Autodesk Inventor part; units mm, degrees
ref_plane "YZ Plane" through (0, 0, 0) normal (1, 0, 0) x (0, 1, 0)
ref_plane "XZ Plane" through (0, 0, 0) normal (0, 1, 0) x (-1, 0, 0)
ref_plane "XY Plane" through (0, 0, 0) normal (0, 0, 1) x (1, 0, 0)
sketch "Esquisse1" plane through (0, 0, 0) normal (0, 1, 0) x (-1, 0, 0)
  circle A0 centre (0, 0) radius 12.5
  dimension "d0" = 25
extrude "Extrusion1" add sketch "Esquisse1" along normal blind 2
sketch "Esquisse2" plane through (0, 2, 0) normal (0, 1, 0) x (1, 0, 0)
  circle A0 centre (0, 0) radius 12.5
  circle A1 centre (0, 0) radius 3.5
  dimension "d3" = 7
extrude "Extrusion2" add sketch "Esquisse2" along normal blind 2 contours A1
sketch "Esquisse3" plane through (0, 4, 0) normal (0, 1, 0) x (1, 0, 0)
  circle A0 centre (0, 0) radius 3.5
  circle A1 centre (0, 0) radius 1.5
  line L0 (-1.118, -1) -> (1.118, -1)
  dimension "d6" = 3
  dimension "d7" = 2.5
extrude "Extrusion3" cut sketch "Esquisse3" against normal through all contours A1 L0 picked at (0.0594, -0.1702)
properties part number "Poulie2"
Geometry check sheet. Reference: the model listing, model coordinates, mm. A direction names the side the tool comes from. Round coordinates to 2 decimals unless told otherwise and drop trailing zeros. Write each loop counter-clockwise with the first axis right and the second up, starting at its lowest first coordinate (ties: lowest second). Pieces come first, ordered by that corner, then holes.
Item 1: Go/stop test with flat-tipped pins: pin 1 Ø0.7 at (x, y) = (0, 3) entering from -Z; pin 2 Ø2 at (x, y) = (3.5, 1.5) entering from -Z; pin 3 Ø1.5 at (y, z) = (2.5, 5.5) entering from -X. Record where each tip stops, or that it passes through.
Determined:
pin 1: stops at z = -3.5
pin 2: stops at z = -12.25
pin 3: stops at x = -11.48
Item 2: Section check C-C (y = 3.5). Record the boundary of the cut face in (x, z).
Determined:
outline: circle Ø7 at (0, 0); hole (-1.12, 1) arc R1.5 ccw (long way) to (1.12, 1) - close
Item 3: Material ranges on line 1 along Z through (x, y) = (0, 1.75); line 2 along Z through (x, y) = (0, 2.55); line 3 along Y through (x, z) = (0, -7), recorded low to high.
Determined:
line 1: z = -12.5 to -1.5, 1 to 12.5
line 2: z = -3.5 to -1.5, 1 to 3.5
line 3: y = 0 to 2
Item 4: Section check A-A (x = 0). Record the boundary of the cut face in (y, z), plus the area to 3 significant figures.
Determined:
outline: (0, -12.5) - (2, -12.5) - (2, -3.5) - (4, -3.5) - (4, -1.5) - (0, -1.5) - close; (0, 1) - (4, 1) - (4, 3.5) - (2, 3.5) - (2, 12.5) - (0, 12.5) - close
area: 54.0 mm2
Item 5: Section check B-B (z = 0). Record the boundary of the cut face in (x, y).
Determined:
outline: (-12.5, 0) - (-1.5, 0) - (-1.5, 4) - (-3.5, 4) - (-3.5, 2) - (-12.5, 2) - close; (1.5, 0) - (12.5, 0) - (12.5, 2) - (3.5, 2) - (3.5, 4) - (1.5, 4) - close
Item 6: Section check D-D (x = -10.25). Record the boundary of the cut face in (y, z), plus the area to 3 significant figures.
Determined:
outline: (0, -7.15) - (2, -7.15) - (2, 7.15) - (0, 7.15) - close
area: 28.6 mm2
Item 7: Mould release check, pull along X, two halves, no side actions. Record for faces 1 (the face through (-11.923, 0.986, -3.755)), 2 (the face through (0, 2, 1)), 3 (the face through (-3, 2, -3)): +X half, -X half, draft (parallel to the pull), parting line (faces both ways), or undercut.
Determined:
face 1: parting line
face 2: undercut
face 3: draft
Item 8: Access from +Z, -Z, +X, -X, +Y, -Y to the whole of each face (thin tool, end or side, straight path). Record for faces 4 (the face through (3.233, 2.986, -1.341)), 5 (the face through (0, 0, -3)).
Determined:
face 4: +Y
face 5: +Z, -Z, +X, -X, -Y
